Part print with two shaded views. Sizes in mm from the minimum x, y, z corner. Give positions to 0.01 mm unless a question says otherwise; leave off trailing zeros. Order: outer loops, then holes, each group sorted by start corner. A loop starts at its lowest first (then second) coordinate and runs counter-clockwise, first axis right, second up. Notation, with made-up numbers: (19.5, -17.75) - (48.5, -17.75) arc R19 cw to (48.5, -7.75) - close; hole circle Ø10 at (11.25, -15). An arc over 180 degrees is marked (long way). Return JSON: item names as keys, results as strings. Group by question number.
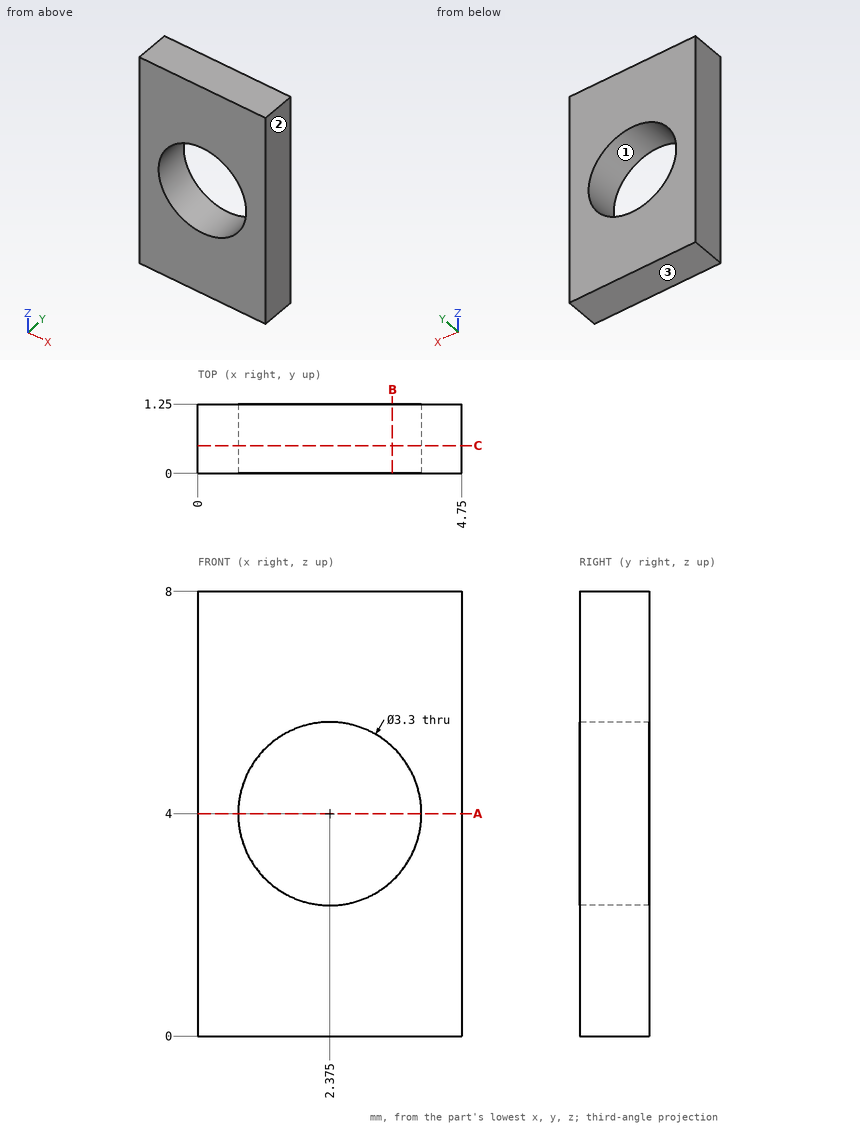
(1) Drill centre lines: L1, parallel to X at y = 0.7, z = 4 (3 decimals); L2, parallel to Z at x = 1.9, y = 0.75; L3, parallel to X at y = 0.6, z = 5.5. Where is each one in solid material? Low to high.
(2) Drop a flat-ended pin along its axis: pin 1 Ø2 at (x, z) = (3.5, 2.5) entering from -Y. Give the stop position or say it passes through.
(3) Pull direction X, two halves, no side cores. Call the marked faces 1, 2 and 3: released by +X, released by -X, zero draft, split by the parting line, or undercut.
(4) Slice it at B-B (x = 3.5). Give the cut face in (y, z), and give its area (3 significant figures).
(5) Slice it at A-A (z = 4). Give the cut face in (x, y) (3 decimals).
(6) Slice it at C-C (y = 0.5). Give the cut face in (x, z) (3 decimals).
Result set:
{
 "1": {"L1": "x = 0 to 0.725, 4.025 to 4.75", "L2": "z = 0 to 2.42, 5.58 to 8", "L3": "x = 0 to 1.69, 3.06 to 4.75"},
 "2": {"pin 1": "stops at y = 0"},
 "3": {"face 1": "undercut", "face 2": "released by +X", "face 3": "zero draft"},
 "4": {"outline": "(0, 0) - (1.25, 0) - (1.25, 2.79) - (0, 2.79) - close; (0, 5.21) - (1.25, 5.21) - (1.25, 8) - (0, 8) - close", "area": "6.98 mm²"},
 "5": {"outline": "(0, 0) - (0.725, 0) - (0.725, 1.25) - (0, 1.25) - close; (4.025, 0) - (4.75, 0) - (4.75, 1.25) - (4.025, 1.25) - close"},
 "6": {"outline": "(0, 0) - (4.75, 0) - (4.75, 8) - (0, 8) - close; hole circle Ø3.3 at (2.375, 4)"}
}
